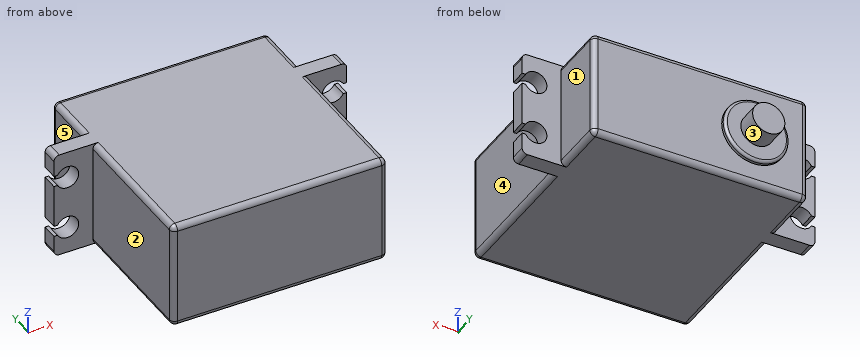
```python
from build123d import *

# Parameters (mm, degrees)
SKETCH1_W           = 40
SKETCH1_H           = 20
BOSS_EXTRUDE1_DEPTH = 40.5
BOSS_EXTRUDE2_DEPTH = 3
FILLET1_R           = 1
SKETCH3_R           = 6
BOSS_EXTRUDE3_DEPTH = 1
SKETCH4_R           = 3
BOSS_EXTRUDE4_DEPTH = 4
FILLET2_R           = 0.5
FILLET3_R           = 1


with BuildPart() as part:
    # Sketch1 → Boss-Extrude1 (new body)
    with BuildSketch(Plane(origin=(0, 0, 0), x_dir=(1, 0, 0), z_dir=(0, 1, 0))):
        Rectangle(SKETCH1_W, SKETCH1_H)
    extrude(amount=BOSS_EXTRUDE1_DEPTH)

    # Sketch2 → Boss-Extrude2 (add)
    with BuildSketch(Plane(origin=(0, 26.8, 0), x_dir=(1, 0, 0), z_dir=(0, 1, 0))):
        with BuildLine():
            Line((-20, -10), (-20, 10))
            Line((-20, 10), (-27.25, 10))
            Line((-27.25, 10), (-27.25, 6))
            Line((-27.25, 6), (-26.596618531, 6))
            ThreePointArc((-26.596618531, 6), (-22.65, 5), (-26.596618531, 4))
            Line((-26.596618531, 4), (-27.25, 4))
            Line((-27.25, 4), (-27.25, -4))
            Line((-27.25, -4), (-26.596618531, -4))
            ThreePointArc((-26.596618531, -4), (-22.65, -5), (-26.596618531, -6))
            Line((-26.596618531, -6), (-27.25, -6))
            Line((-27.25, -6), (-27.25, -10))
            Line((-27.25, -10), (-20, -10))
        make_face()
        with BuildLine():
            Line((27.25, 10), (20, 10))
            Line((20, 10), (20, -10))
            Line((20, -10), (27.25, -10))
            Line((27.25, -10), (27.25, -6))
            Line((27.25, -6), (26.596618531, -6))
            ThreePointArc((26.596618531, -6), (22.65, -5), (26.596618531, -4))
            Line((26.596618531, -4), (27.25, -4))
            Line((27.25, -4), (27.25, 4))
            Line((27.25, 4), (26.596618531, 4))
            ThreePointArc((26.596618531, 4), (22.65, 5), (26.596618531, 6))
            Line((26.596618531, 6), (27.25, 6))
            Line((27.25, 6), (27.25, 10))
        make_face()
    extrude(amount=BOSS_EXTRUDE2_DEPTH)

    # Fillet1
    fillet1_edges = [part.edges().sort_by_distance(p)[0] for p in [
        (-27.25, 28.3, 10),
        (-27.25, 28.3, -10),
        (27.25, 28.3, -10),
        (27.25, 28.3, 10),
    ]]
    fillet(fillet1_edges, radius=FILLET1_R)

    # Sketch3 → Boss-Extrude3 (add)
    with BuildSketch(Plane(origin=(0, 40.5, 0), x_dir=(1, 0, 0), z_dir=(0, 1, 0))):
        with Locations((-10, 0)):
            Circle(SKETCH3_R)
    extrude(amount=BOSS_EXTRUDE3_DEPTH)

    # Sketch4 → Boss-Extrude4 (add)
    with BuildSketch(Plane(origin=(0, 41.5, 0), x_dir=(1, 0, 0), z_dir=(0, 1, 0))):
        with Locations((-10, 0)):
            Circle(SKETCH4_R)
    extrude(amount=BOSS_EXTRUDE4_DEPTH)

    # Fillet2
    fillet2_edges = [part.edges().sort_by_distance(p)[0] for p in [
        (-16, 41.5, 0),
    ]]
    fillet(fillet2_edges, radius=FILLET2_R)

    # Fillet3
    fillet3_edges = [part.edges().sort_by_distance(p)[0] for p in [
        (-20, 40.5, 0),
        (0, 40.5, 10),
        (-20, 13.4, 10),
        (-20, 13.4, -10),
        (20, 13.4, -10),
        (20, 13.4, 10),
        (20, 40.5, 0),
        (0, 0, 10),
        (-20, 0, 0),
        (0, 0, -10),
        (20, 0, 0),
        (0, 40.5, -10),
        (20, 35.15, 10),
        (-20, 35.15, 10),
        (-20, 35.15, -10),
        (20, 35.15, -10),
    ]]
    fillet(fillet3_edges, radius=FILLET3_R)


solid = part.part
```
Verification items for the finished model (mm, model axes). Face numbers are marked on the shaded views. A direction names the side the tool comes from. Coordinates: 2 decimals unless noted, no trailing zeros. Write each loop counter-clockwise with the first axis right and the second up, starting at its lowest first coordinate (ties: lowest second). Pieces come first, ordered by that corner, then holes. Notation, with made-up numbers: M -13.5,-30.5 L 11.5,-30.5 A32 ccw 11.5,-3.5 Z; hole C -32.5,-25 d1. An arc over 180 degrees is marked long. Answer as a JSON object with one key per item and string values. Group by question number.
(1) Material ranges on line 1 (Z direction, x = -24.75, y = 28.35); line 2 (Z direction, x = 24, y = 27); line 3 (X direction, y = 6, z = 6), recorded low to high.
(2) Gauge pin test, flat ends, axial feed: pin 1 (0.7 mm diameter, centred on x = -27, y = 28.5, fed in from -Z); pin 2 (0.5 mm diameter, centred on x = -27, y = 28.5, fed in from +Z); pin 3 (12 mm diameter, centred on y = 8, z = 5, fed in from -X). Record the tip position at first contact, or that the pin passes through.
(3) Cross-section at B-B, the plane y = 33. Record the cut outline in (x, z).
(4) Tool access check on the marked faces 1, 2, 3, 4 and 5. Record the directions out of +Z, -Z, +X, -X, +Y, -Y that give a thin tool (end or side, any length) a straight path to the whole face; none if there is none.
(5) Cross-section at A-A, the plane x = 24.75. Record the cut outline in (y, z), and give its area (3 significant figures).
(6) Cross-section at C-C, the plane x = 10.5. Record the cut outline in (y, z), and give its area (3 significant figures).
(7) Cross-section at D-D, the plane z = 0. Record the cut outline in (x, y).
Reply:
{
 "1": {"line 1": "-10 to -7.1, -2.9 to 2.9, 7.1 to 10", "line 2": "-10 to -6.96, -3.04 to 3.04, 6.96 to 10", "line 3": "-20 to 20"},
 "2": {"pin 1": "z = -9.92", "pin 2": "z = 9.87", "pin 3": "x = -20"},
 "3": {"outline": "M -20,-9 A1 ccw -19,-10 L 19,-10 A1 ccw 20,-9 L 20,9 A1 ccw 19,10 L -19,10 A1 ccw -20,9 Z"},
 "4": {"face 1": "+Z, -Z, +X, +Y", "face 2": "+Z, -Z, -X, -Y", "face 3": "+Y", "face 4": "+Z, -Z, +X, -Y", "face 5": "+Z, -Z, -X, +Y"},
 "5": {"outline": "M 26.8,-10 L 29.8,-10 L 29.8,-7.1 L 26.8,-7.1 Z; M 26.8,-2.9 L 29.8,-2.9 L 29.8,2.9 L 26.8,2.9 Z; M 26.8,7.1 L 29.8,7.1 L 29.8,10 L 26.8,10 Z", "area": "34.8 mm²"},
 "6": {"outline": "M 0,-9 A1 ccw 1,-10 L 39.5,-10 A1 ccw 40.5,-9 L 40.5,9 A1 ccw 39.5,10 L 1,10 A1 ccw 0,9 Z", "area": "809 mm²"},
 "7": {"outline": "M -27.25,26.8 L -20,26.8 L -20,1 A1 ccw -19,0 L 19,0 A1 ccw 20,1 L 20,26.8 L 27.25,26.8 L 27.25,29.8 L 20,29.8 L 20,39.5 A1 ccw 19,40.5 L -4,40.5 L -4,41 A0.5 ccw -4.5,41.5 L -7,41.5 L -7,45.5 L -13,45.5 L -13,41.5 L -15.5,41.5 A0.5 ccw -16,41 L -16,40.5 L -19,40.5 A1 ccw -20,39.5 L -20,29.8 L -27.25,29.8 Z"}
}
